Work out the finished part from the listing and answer in its coordinate system (mm). Face numbers are marked on the shaded views. A direction names the side the tool comes from. Round coordinates to 2 decimals unless told otherwise and drop trailing zeros. Loops run counter-clockwise (first coordinate to the right, second up) from the corner with the lowest first, then second, coordinate; pieces in that order, holes last. Notation, with made-up numbers: (72.25, 64.25) -> (110.25, 64.25) arc R18 ccw to (110.25, 79.25) -> close; hole circle Ø7 at (81, -16). An arc over 180 degrees is marked (long way). Use one line per item in the form item = value.
Autodesk Inventor part; units mm, degrees
ref_plane "YZ Plane" through (0, 0, 0) normal (1, 0, 0) x (0, 1, 0)
ref_plane "XZ Plane" through (0, 0, 0) normal (0, 1, 0) x (-1, 0, 0)
ref_plane "XY Plane" through (0, 0, 0) normal (0, 0, 1) x (1, 0, 0)
sketch "Sketch1" plane through (0, 0, 0) normal (0, 0, 1) x (1, 0, 0)
  line L0 (0, 0) -> (241.3, 0)
  line L1 (241.3, 0) -> (241.3, 60.96)
  line L2 (241.3, 60.96) -> (0, 60.96)
  line L3 (0, 60.96) -> (0, 0)
  dimension "d0" = 241.3
  dimension "d1" = 60.96
extrude "Extrusion1" add sketch "Sketch1" along normal blind 3.175
sketch "Sketch2" plane through (0, 0, 0) normal (0, 0, -1) x (-1, 0, 0)
  line L0 (-241.3, 60.96) -> (0, 60.96)
  line L1 (-241.3, 0) -> (-241.3, 60.96)
  line L2 (0, 60.96) -> (-241.3, 60.96)
  line L3 (-241.3, 60.96) -> (-241.3, 56.1975)
  line L4 (-241.3, 56.1975) -> (0, 56.1975)
  line L5 (0, 56.1975) -> (0, 60.96)
  point P0 (0, 0)
  dimension "d4" = 4.7625
extrude "Extrusion2" add sketch "Sketch2" along normal blind 23.495
sketch "Sketch3" plane through (0, 60.96, 3.175) normal (0, 1, 0) x (1, 0, 0)
  circle A0 centre (38.1, 14.2875) radius 3.0988
  circle A1 centre (215.9, 14.2875) radius 3.0988
  line L0 (241.3, 26.67) -> (241.3, 0)
  line L1 (0, 26.67) -> (241.3, 26.67)
  point P0 (0, 3.175)
  dimension "d7" = 6.1976
  dimension "d8" = 6.1976
  dimension "d9" = 177.8
  dimension "d10" = 25.4
  dimension "d11" = 12.3825
  dimension "d12" = 12.3825
extrude "Extrusion3" cut sketch "Sketch3" against normal blind 6.1976
equation "\"d12\" = d11"
equation "\"d13\" = d8"
properties part number "Camera Mount"
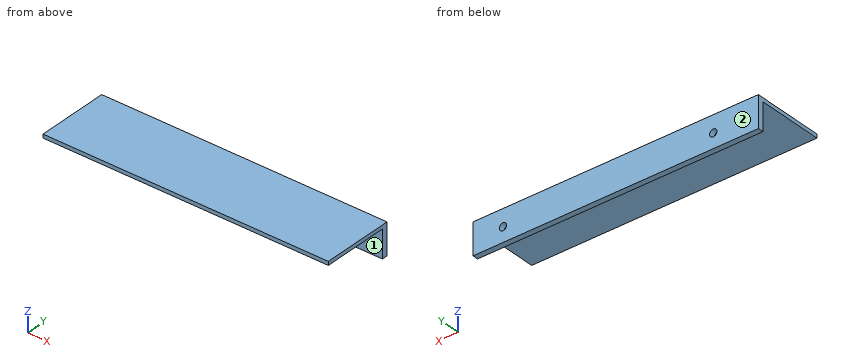
(1) Consider L1, parallel to Z at x = 38, y = 59 (3 decimals); L2, parallel to Y at x = 168.5, z = -17.75; L3, parallel to Z at x = 40, y = 19.5 (3 decimals). Determine where each line is inside the solid, lowest interval first.
Completed:
L1 = -23.495 to -14.21, -8.015 to 3.175
L2 = 56.2 to 60.96
L3 = 0 to 3.175
(2) Find section D-D, the plane z = -2.5. Write down the section's boundary in (x, y).
Completed:
outline = (0, 56.2) -> (241.3, 56.2) -> (241.3, 60.96) -> (0, 60.96) -> close
(3) Given P1, Ø10, axis at x = 57.5, z = -15, coming from the -Y side; P2, Ø3, axis at x = 138, y = 15.5, coming from the -Z side, each flat-ended and moving along its own axis, determine where each tip first touches the part or whether it passes through.
Completed:
P1 = 56.2
P2 = 0
(4) For the marked faces 1 and 2, determine the directions among +Z, -Z, +X, -X, +Y, -Y from which every point of the face is accessible in a straight line to the end or side of a thin tool.
Completed:
face_1 = -Z, +X, -X, -Y
face_2 = +Z, -Z, +X, -X, +Y
(5) Find section C-C, the plane x = 89. Write down the section's boundary in (y, z) (1 decimal), then the cut area to 3 significant figures.
Completed:
outline = (0, 0) -> (56.2, 0) -> (56.2, -23.5) -> (61, -23.5) -> (61, 3.2) -> (0, 3.2) -> close
area = 305 mm2
(6) Find section A-A, the plane x = 38.1. Write down the section's boundary in (y, z) (1 decimal), then the cut area to 3 significant figures.
Completed:
outline = (0, 0) -> (56.2, 0) -> (56.2, -8) -> (61, -8) -> (61, 3.2) -> (0, 3.2) -> close; (56.2, -23.5) -> (61, -23.5) -> (61, -14.2) -> (56.2, -14.2) -> close
area = 276 mm2
(7) Find section B-B, the plane y = 16. Write down the section's boundary in (x, z) (3 decimals), then the cut area to 3 significant figures.
Completed:
outline = (0, 0) -> (241.3, 0) -> (241.3, 3.175) -> (0, 3.175) -> close
area = 766 mm2
